Verification items for the finished model (mm, model axes). A direction names the side the tool comes from. Coordinates: 2 decimals unless noted, no trailing zeros. Loops run counter-clockwise (first coordinate to the right, second up) from the corner with the lowest first, then second, coordinate; pieces in that order, holes last. Notation, with made-up numbers: (19, 52.5) -> (33, 52.5) arc R12 cw to (33, 69.5) -> close; hole circle Ø7 at (-10.5, 5). An arc over 180 degrees is marked (long way). Answer as a JSON object with one key per item and string values. Group by question number.
Q1. Cross-section at C-C on x = -10.5. Record the boundary of the cut face in (y, z), and give its area (3 significant figures).
Q2. Gauge pin test, flat ends, axial feed: pin 1 Ø2 at (x, z) = (-1.5, 100) entering from -Y; pin 2 Ø15 at (x, z) = (6, 116) entering from -Y; pin 3 Ø8 at (x, z) = (-12, 110) entering from +Y; pin 4 Ø12 at (y, z) = (14.5, 85) entering from -X. Record the tip position at first contact, or that the pin passes through.
Q3. Cross-section at A-A on z = 5. Record the boundary of the cut face in (x, y).
Q4. Scan lines: L1, parallel to X at y = -3.9, z = 5; L2, parallel to X at y = 19.5, z = 94.5; L3, parallel to Y at x = 10, z = 37. Record each from-to range of solid material in increasing order.
Q5. Cross-section at D-D on z = 61. Record the boundary of the cut face in (x, y), and give its area (3 significant figures).
Q6. Set-up check for faces 4 (the cylindrical face through (1.3, 31.8, 114.5)), 5 (the flat face through (-11, -5, 20)): record each of +Z, -Z, +X, -X, +Y, -Y from which the full face is reachable in a straight line by a thin tool's end or side.
Q7. Release check for a two-part mould opening along Y. For faces 1 (the flat face through (-16.146, -5.197, 17.535)), 2 (the flat face through (-1, 23.775, 115.5)), 3 (the flat face through (1, 30.275, 115)) record: released by +Y, released by -Y, zero draft, split by the parting line, or undercut.
Q8. Cross-section at B-B on z = 113. Record the boundary of the cut face in (x, y).
Autodesk Inventor part; units mm, degrees
ref_plane "YZ Plane" through (0, 0, 0) normal (1, 0, 0) x (0, 1, 0)
ref_plane "XZ Plane" through (0, 0, 0) normal (0, 1, 0) x (-1, 0, 0)
ref_plane "XY Plane" through (0, 0, 0) normal (0, 0, 1) x (1, 0, 0)
sketch "Sketch1" plane through (0, 0, 0) normal (0, 0, 1) x (1, 0, 0)
  line L0 (-18.6815, -3.2252) -> (11.3185, -3.2252)
  line L1 (11.3185, -3.2252) -> (11.3185, -7.2252)
  line L2 (11.3185, -7.2252) -> (-18.6815, -7.2252)
  line L3 (-18.6815, -7.2252) -> (-18.6815, -3.2252)
  point P0 (0, 0)
  dimension "d0" = 30
  dimension "d1" = 4
extrude "Extrusion1" add sketch "Sketch1" along normal blind 20
sketch "Sketch2" plane through (-18.6815, -7.2252, 0) normal (0, -1, 0) x (1, 0, 0)
  line L0 (30, 20) -> (10, 20)
  line L1 (10, 20) -> (10, 123)
  line L2 (10, 123) -> (30, 123)
  line L3 (30, 123) -> (30, 20)
  point P0 (18.6815, 0)
  dimension "d4" = 103
  dimension "d5" = 20
extrude "Extrusion2" add sketch "Sketch2" against normal blind 10
sketch "Sketch3" plane through (-18.6815, -7.2252, 0) normal (0, -1, 0) x (1, 0, 0)
  line L0 (30, 20) -> (10, 20)
  line L1 (30, 0) -> (30, 20)
  line L2 (30, 0) -> (0, 0)
  point P0 (18.6815, 0)
  point P1 (25, 15)
  point P2 (25, 5)
  point P3 (15, 5)
  dimension "d8" = 5
  dimension "d9" = 5
  dimension "d10" = 5
  dimension "d11" = 5
  dimension "d12" = 5
  dimension "d13" = 10
hole "Hole1" at (6.3185, -7.2252, 15) at (6.3185, -7.2252, 5) at (-3.6815, -7.2252, 5) direction (0, 1, 0) diameter 3 depth 8 tip angle 118 countersink diameter 6 countersink angle 90
chamfer "Chamfer1" distance 5 angle 45 1 edges at (-18.6815, -5.2252, 20)
sketch "Sketch4" plane through (-8.6815, -7.2252, 20) normal (-1, 0, 0) x (0, 0, 1)
  line L0 (103, 10) -> (0, 10)
  line L1 (0, 10) -> (0, 4)
  line L2 (0, 4) -> (103, 4)
  line L3 (103, 4) -> (103, 10)
  point P0 (-20, 7.2252)
extrude "Extrusion3" cut sketch "Sketch4" against normal blind 20
sketch "Sketch5" plane through (-8.6815, -7.2252, 20) normal (-1, 0, 0) x (0, 0, 1)
  line L0 (103, 4) -> (99, 4)
  line L1 (99, 4) -> (99, 34)
  line L2 (99, 34) -> (103, 34)
  line L3 (103, 34) -> (103, 4)
  point P0 (-20, 7.2252)
  dimension "d26" = 4
  dimension "d27" = 30
extrude "Extrusion4" add sketch "Sketch5" against normal blind 20
sketch "Sketch6" plane through (-8.6815, -7.2252, 20) normal (-1, 0, 0) x (0, 0, 1)
  line L0 (103, 34) -> (88, 34)
  line L1 (88, 34) -> (88, 31)
  line L2 (88, 31) -> (103, 31)
  line L3 (103, 31) -> (103, 34)
  line L4 (103, 37.5) -> (88, 37.5)
  line L5 (88, 37.5) -> (88, 40.5)
  line L6 (88, 40.5) -> (103, 40.5)
  line L7 (103, 40.5) -> (103, 37.5)
  line L8 (103, 0) -> (103, 34)
  line L9 (88, 40.5) -> (84, 40.5)
  line L10 (84, 40.5) -> (84, 31)
  line L11 (84, 31) -> (88, 31)
  line L12 (88, 31) -> (88, 40.5)
  point P0 (-20, 7.2252)
  dimension "d30" = 15
  dimension "d31" = 3
  dimension "d32" = 3.5
  dimension "d33" = 3
  dimension "d34" = 4
extrude "Extrusion5" add sketch "Sketch6" against normal blind 20
sketch "Sketch7" plane through (-8.6815, -7.2252, 20) normal (-1, 0, 0) x (0, 0, 1)
  line L0 (88, 37.5) -> (87, 37.5)
  line L1 (87, 37.5) -> (87, 34)
  line L2 (87, 34) -> (88, 34)
  line L3 (88, 34) -> (88, 37.5)
  line L4 (103, 34) -> (88, 34)
  point P0 (-20, 7.2252)
  dimension "d37" = 1
extrude "Extrusion6" cut sketch "Sketch7" against normal blind 20
sketch "Sketch8" plane through (-8.6815, -7.2252, 20) normal (-1, 0, 0) x (0, 0, 1)
  line L0 (103, 34) -> (103, 0)
  line L1 (-20, 0) -> (103, 0)
  line L2 (103, 31) -> (50, 31)
  line L3 (50, 31) -> (50, 0)
  line L4 (50, 0) -> (103, 0)
  line L5 (103, 0) -> (103, 31)
  line L6 (84, 31) -> (99, 31)
  line L7 (0, 0) -> (0, 4)
  point P0 (-20, 7.2252)
  dimension "d40" = 50
extrude "Extrusion7" cut sketch "Sketch8" against normal blind 20
sketch "Sketch9" plane through (11.3185, -7.2252, 0) normal (1, 0, 0) x (0, 0, -1)
  line L0 (-104, 40.5) -> (-104, 31)
  line L1 (-104, 31) -> (-104, 40.5)
  line L2 (-104, 31) -> (-70, 0)
  line L3 (-104, 40.5) -> (-70, 9.5)
  line L4 (-70, 9.5) -> (-70, 0)
  line L5 (-70, 4) -> (-70, 0)
  line L6 (-70, 9.5) -> (-59.5806, 0)
  line L7 (-59.5806, 0) -> (-70, 0)
  line L8 (0, 0) -> (-70, 0)
  point P0 (0, 7.2252)
extrude "Extrusion8" add sketch "Sketch9" against normal blind 20
sketch "Sketch10" plane through (-8.6815, 23.7748, 123) normal (0, -1, 0) x (1, 0, 0)
  line L0 (0, -16) -> (20, -16)
  point P0 (8.6815, -123)
  point P1 (10, -10)
  dimension "d45" = 6
hole "Hole2" at (1.3185, 23.7748, 113) direction (0, 1, 0) diameter 3 depth 15 tip angle 118 countersink diameter 6 countersink angle 90
chamfer "Chamfer2" distance 5.5 angle 45 4 edges at (11.3185, 31.7748, 123) (-8.6815, 31.7748, 123) (11.3185, 25.2748, 123) (-8.6815, 25.2748, 123)
properties part number "col support base"
Computed values:
{
 "1": {"outline": "(-7.23, 0) -> (-3.23, 0) -> (-3.23, 20) -> (-7.23, 20) -> close", "area": "80.0 mm²"},
 "2": {"pin 1": "stops at y = 19.22", "pin 2": "stops at y = 23.77", "pin 3": "stops at y = 33.27", "pin 4": "stops at x = -8.68"},
 "3": {"outline": "(-18.68, -7.23) -> (-6.68, -7.23) -> (-5.18, -5.73) -> (-5.18, -3.23) -> (-18.68, -3.23) -> close; (-2.18, -5.73) -> (-0.68, -7.23) -> (3.32, -7.23) -> (4.82, -5.73) -> (4.82, -3.23) -> (-2.18, -3.23) -> close; (7.82, -5.73) -> (9.32, -7.23) -> (11.32, -7.23) -> (11.32, -3.23) -> (7.82, -3.23) -> close"},
 "4": {"L1": "x = -18.68 to -5.18, -2.18 to 4.82, 7.82 to 11.32", "L2": "x = -8.68 to 11.32", "L3": "y = -7.23 to -3.23"},
 "5": {"outline": "(-8.68, -7.23) -> (11.32, -7.23) -> (11.32, -3.23) -> (-8.68, -3.23) -> close", "area": "80.0 mm²"},
 "6": {"face 4": "+Y, -Y", "face 5": "+Z, -X, +Y, -Y"},
 "7": {"face 1": "zero draft", "face 2": "released by -Y", "face 3": "undercut"},
 "8": {"outline": "(-8.68, 23.77) -> (-1.68, 23.77) -> (-0.18, 25.27) -> (-0.18, 26.77) -> (-8.68, 26.77) -> close; (-8.68, 30.27) -> (-0.18, 30.27) -> (-0.18, 33.27) -> (-8.68, 33.27) -> close; (2.82, 25.27) -> (4.32, 23.77) -> (11.32, 23.77) -> (11.32, 26.77) -> (2.82, 26.77) -> close; (2.82, 30.27) -> (11.32, 30.27) -> (11.32, 33.27) -> (2.82, 33.27) -> close"}
}
